```python
from build123d import *

# Parameters (mm, degrees)
SKETCH1_R             = 1.7
BOSS_EXTRUDE1_DEPTH   = 5
BOSS_EXTRUDE1_2_DEPTH = 5
SKETCH2_R             = 1.7
BOSS_EXTRUDE5_DEPTH   = 2.5
SKETCH3_R             = 1.2
BOSS_EXTRUDE6_DEPTH   = 2.5
SKETCH4_R             = 1.7
BOSS_EXTRUDE7_DEPTH   = 5


with BuildPart() as part:
    # Sketch1 → Boss-Extrude1 (new body)
    with BuildSketch(Plane(origin=(0, 0, 0), x_dir=(1, 0, 0), z_dir=(0, 1, 0))):
        with Locations(Location((0, 0, 0), (0, 0, 270))):
            Circle(SKETCH1_R)
    extrude(amount=BOSS_EXTRUDE1_DEPTH)



with BuildPart() as body_2:
    # Sketch1 → Boss-Extrude1 2 (new body)
    with BuildSketch(Plane(origin=(0, 0, 0), x_dir=(1, 0, 0), z_dir=(0, 1, 0))):
        with Locations(Location((70, 0, 0), (0, 0, 270))):
            Circle(SKETCH1_R)
    extrude(amount=BOSS_EXTRUDE1_2_DEPTH)


with BuildPart() as part_1:
    add(part.part)

    add(body_2.part)  # Boss-Extrude5 merges body 2
    # Sketch2 → Boss-Extrude5 (add)
    # profile 1 of 4: a face of its own
    with BuildSketch(Plane(origin=(0, 5, 0), x_dir=(1, 0, 0), z_dir=(0, 1, 0))):
        with BuildLine():
            ThreePointArc((-1.889706262, 2.826483725), (-0.987409575, 3.253463129), (0, 3.4))
            Line((0, 3.4), (11.202822944, 3.4))
            Line((11.202822944, 3.4), (35, 19.310112661))
            Line((35, 19.310112661), (35, 23.4))
            Line((35, 23.4), (35, 26.8))
            ThreePointArc((35, 26.8), (34.012590425, 26.653463129), (33.110293738, 26.226483725))
            Line((33.110293738, 26.226483725), (-1.889706262, 2.826483725))
        make_face()
    # profile 2 of 4: a face of its own
    with BuildSketch(Plane(origin=(0, 5, 0), x_dir=(1, 0, 0), z_dir=(0, 1, 0))):
        with BuildLine():
            Line((0, -3.4), (70, -3.4))
            ThreePointArc((70, -3.4), (73.4, 0), (70, 3.4))
            Line((70, 3.4), (0, 3.4))
            ThreePointArc((0, 3.4), (-3.4, 0), (0, -3.4))
        make_face()
        with Locations(Location((10, 0, 0), (0, 0, 270))):
            Circle(SKETCH2_R, mode=Mode.SUBTRACT)
        with Locations(Location((60, 0, 0), (0, 0, 270))):
            Circle(SKETCH2_R, mode=Mode.SUBTRACT)
        with Locations(Location((0, 0, 0), (0, 0, 270))):
            Circle(SKETCH2_R, mode=Mode.SUBTRACT)
    # profile 3 of 4: a face of its own
    with BuildSketch(Plane(origin=(0, 5, 0), x_dir=(1, 0, 0), z_dir=(0, 1, 0))):
        with Locations(Location((0, 0, 0), (0, 0, 270))):
            Circle(SKETCH2_R)
    # profile 4 of 4: a face of its own
    with BuildSketch(Plane(origin=(0, 5, 0), x_dir=(1, 0, 0), z_dir=(0, 1, 0))):
        with BuildLine():
            Line((35, 23.4), (35, 19.310112661))
            Line((35, 19.310112661), (58.797177056, 3.4))
            Line((58.797177056, 3.4), (70, 3.4))
            ThreePointArc((70, 3.4), (70.987409575, 3.253463129), (71.889706262, 2.826483725))
            Line((71.889706262, 2.826483725), (36.889706262, 26.226483725))
            ThreePointArc((36.889706262, 26.226483725), (35.987409575, 26.653463129), (35, 26.8))
            Line((35, 26.8), (35, 23.4))
        make_face()
    extrude(amount=BOSS_EXTRUDE5_DEPTH)

    # Sketch3 → Boss-Extrude6 (add)
    with BuildSketch(Plane.XZ):
        with Locations(Location((0, 0, 0), (0, 0, 270))):
            Circle(SKETCH3_R)
        with Locations(Location((70, 0, 0), (0, 0, 270))):
            Circle(SKETCH3_R)
    extrude(amount=BOSS_EXTRUDE6_DEPTH)

    # Sketch4 → Boss-Extrude7 (add)
    with BuildSketch(Plane.XZ.offset(-5)):
        with Locations(Location((35, -23.4, 0), (0, 0, 90))):
            Circle(SKETCH4_R)
    extrude(amount=BOSS_EXTRUDE7_DEPTH)


solid = part_1.part
```
Source: CAD feature listing. Evaluate the final solid. Frame: model axes, mm. A direction names the side the tool comes from. Coordinates: 2 decimals unless noted, no trailing zeros. Loops run counter-clockwise (first coordinate to the right, second up) from the corner with the lowest first, then second, coordinate; pieces in that order, holes last. Notation, with made-up numbers: M 35.5,72 L 72.5,72 A5 ccw 72.5,79 Z; hole C 67.25,19.25 d11. An arc over 180 degrees is marked long. Use CSV: the item, a comma, the result in double quotes.
(1) Cut plane A-A on z = 0. Return loops of the section in (x, y).
Answers follow:
outline,"M -3.4,5 L -1.7,5 L -1.7,0 L -1.2,0 L -1.2,-2.5 L 1.2,-2.5 L 1.2,0 L 1.7,0 L 1.7,5 L 8.3,5 L 8.3,7.5 L -3.4,7.5 Z; M 11.7,5 L 58.3,5 L 58.3,7.5 L 11.7,7.5 Z; M 61.7,5 L 68.3,5 L 68.3,0 L 68.8,0 L 68.8,-2.5 L 71.2,-2.5 L 71.2,0 L 71.7,0 L 71.7,5 L 73.4,5 L 73.4,7.5 L 61.7,7.5 Z"
(2) Draft query along X for faces 4 (the face through (61.686, 6.232, -0.221)), 5 (the face through (0, -2.5, 0)), 6 (the face through (-3.27, 6.23, 0.93)). Return one class per face: pulls with the +X half, pulls with the -X half, needs draft (parallel to the pull), parting line crosses it, or undercut.
Answers follow:
face 4,"undercut"
face 5,"needs draft"
face 6,"pulls with the -X half"
(3) Cut plane B-B on x = 17. Return loops of the section in (y, z), and give its area (3 significant figures).
Answers follow:
outline,"M 5,-15.46 L 7.5,-15.46 L 7.5,-7.28 L 5,-7.28 Z; M 5,-3.4 L 7.5,-3.4 L 7.5,3.4 L 5,3.4 Z"
area,"37.4 mm²"
(4) Cut plane C-C on y = 1. Return loops of the section in (x, z), and give its area (3 significant figures).
Answers follow:
outline,"C 0,0 d3.4; C 35,-23.4 d3.4; C 70,0 d3.4"
area,"27.2 mm²"
(5) Cut plane D-D on z = -14. Return loops of the section in (x, y), and give its area (3 significant figures).
Answers follow:
outline,"M 14.82,5 L 27.06,5 L 27.06,7.5 L 14.82,7.5 Z; M 42.94,5 L 55.18,5 L 55.18,7.5 L 42.94,7.5 Z"
area,"61.2 mm²"
(6) Line query: line 1 (X direction, y = 6.6, z = 0); line 2 (Y direction, x = 23, z = 0.5); line 3 (Y direction, x = 69, z = 1). Output: solid intervals per line, ascending. Write a range as [from, to].
Answers follow:
line 1,"[-3.4, 8.3], [11.7, 58.3], [61.7, 73.4]"
line 2,"[5, 7.5]"
line 3,"[0, 7.5]"
(7) Reachability of faces 1 (the face through (35, 6, -3.4)), 2 (the face through (15.855, 6.232, -14.69)), 3 (the face through (71.19, -1.23, 0.16)) from +Z, -Z, +X, -X, +Y, -Y: full face, straight path, thin tool, end or side. Return the list, or none.
Answers follow:
face 1,"+Y, -Y"
face 2,"-Z, -X, +Y, -Y"
face 3,"-Y"
(8) Contact query for flat-ended pins moving along their axis: pin 1 (10 mm diameter, centred on x = 47, z = -17, fed in from -Y); pin 2 (2 mm diameter, centred on x = 38.5, y = 6.5, fed in from -Z); pin 3 (1 mm diameter, centred on y = 6, z = -13, fed in from +X). Output: stop coordinate, or through.
Answers follow:
pin 1,"y = 5"
pin 2,"z = -25.82"
pin 3,"x = 57.42"
